The drawing under review shows one solid part. Ordinate dimensions are in mm from its lowest x, y, z. A direction names the side the tool comes from. Coordinates: 2 decimals unless noted, no trailing zeros. Write each loop counter-clockwise with the first axis right and the second up, starting at its lowest first coordinate (ties: lowest second). Pieces come first, ordered by that corner, then holes.
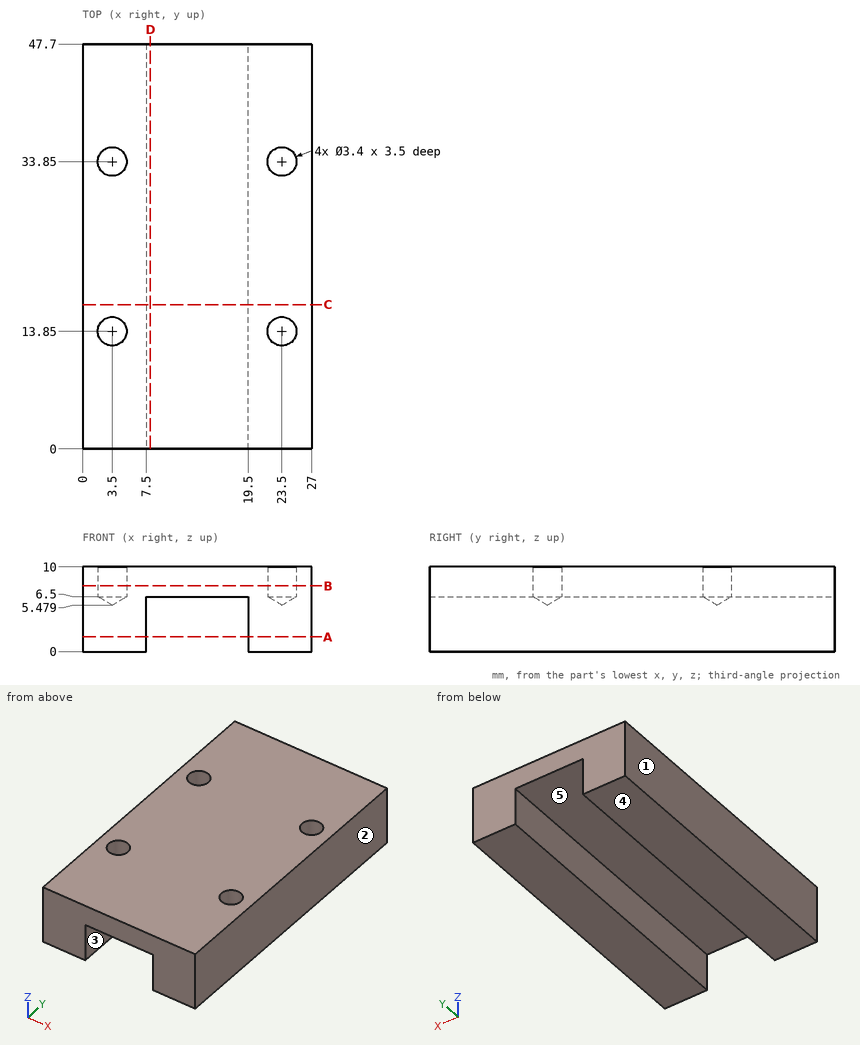
Q1. Add section A-A (z = 1.75). State the section outline as (x, y) points.
Ans:
outline: (0, 0) - (7.5, 0) - (7.5, 47.7) - (0, 47.7) - close; (19.5, 0) - (27, 0) - (27, 47.7) - (19.5, 47.7) - close
Q2. For probe 1 along Y at (x, z) = (23.5, 8.25); probe 2 along X at (y, z) = (33.85, 8.6); probe 3 along X at (y, z) = (3.5, 4.5), list the stretches that pass through material, from the lowest coordinate up.
Ans:
probe 1: y = 0 to 12.15, 15.55 to 32.15, 35.55 to 47.7
probe 2: x = 0 to 1.8, 5.2 to 21.8, 25.2 to 27
probe 3: x = 0 to 7.5, 19.5 to 27
Q3. Draft analysis for pull direction X (two halves, no side actions). For the marked faces 1, 2 and 3, state which applies: +X half, -X half, draft (parallel to the pull), parting line (faces both ways), or undercut.
Ans:
face 1: -X half
face 2: +X half
face 3: undercut
Q4. Clearance check with a flat-ended pin moving along its axis: pin 1 Ø2.5 at (x, y) = (3.5, 33.85) entering from +Z. State where the tip first meets the part, or that it passes through.
Ans:
pin 1: stops at z = 6.23
Q5. Add section D-D (x = 8). State the section outline as (y, z) points.
Ans:
outline: (0, 6.5) - (47.7, 6.5) - (47.7, 10) - (0, 10) - close
Q6. Add section C-C (y = 17). State the section outline as (x, z) points.
Ans:
outline: (0, 0) - (7.5, 0) - (7.5, 6.5) - (19.5, 6.5) - (19.5, 0) - (27, 0) - (27, 10) - (0, 10) - close
Q7. Add section B-B (z = 7.75). State the section outline as (x, y) points.
Ans:
outline: (0, 0) - (27, 0) - (27, 47.7) - (0, 47.7) - close; hole circle Ø3.4 at (3.5, 13.85); hole circle Ø3.4 at (3.5, 33.85); hole circle Ø3.4 at (23.5, 13.85); hole circle Ø3.4 at (23.5, 33.85)
Q8. Tool access review of the marked faces 4 and 5: name each direction out of +Z, -Z, +X, -X, +Y, -Y from which nothing blocks a thin tool from reaching the whole face with its end or side.
Ans:
face 4: -Z, +X, -X, +Y, -Y
face 5: -Z, +Y, -Y
